Check sheet for the modelled part. Datum: model origin and axes. Units: mm. A direction names the side the tool comes from. Give positions to 0.01 mm unless a question says otherwise; leave off trailing zeros. Loops run counter-clockwise (first coordinate to the right, second up) from the corner with the lowest first, then second, coordinate; pieces in that order, holes last. Notation, with made-up numbers: (28.5, -6) - (82.5, -6) arc R16 ccw to (82.5, 8) - close; hole circle Ø3 at (-34.5, -0.75). An arc over 180 degrees is marked (long way). Answer in a Markdown table with one row per item. Add a question column.
(1) Thickness scan on L1, parallel to Y at x = 53.2, z = 1.15; L2, parallel to Z at x = 58.5, y = -27.4; L3, parallel to Z at x = 52.5, y = -24.5. Record the ranges inside material, lowest first.
(2) Sectioned sample at D-D on y = -27. Enter the section's corners in (x, z).
(3) Sectioned sample at A-A on x = 53.2. Enter the section's corners in (y, z), then the cut area to 3 significant figures.
(4) Set-up check for faces 4 (the face through (54, -10, 3)), 5 (the face through (55.2, 4, 8)), 6 (the face through (58, -20.162, 31)), 7 (the face through (59, -24.661, 40)): record each of +Z, -Z, +X, -X, +Y, -Y from which the full face is reachable in a straight line by a thin tool's end or side.
(5) Draft check along X on faces 1 (the face through (55.2, -22, 52)), 2 (the face through (58.242, -7.389, 47.625)), 3 (the face through (54.38, 2.98, 1.48)). Enter one of: released by +X, released by -X, zero draft, split by the parting line, or undercut.
(6) Go/stop test with flat-tipped pins: P1, Ø6, axis at x = 57, z = 77, coming from the -Y side; P2, Ø6.5, axis at x = 58, z = 27.5, coming from the +Y side; P3, Ø0.8, axis at y = 4, z = 10, coming from the -X side. Record where each tip stops, or that it passes through.
(7) Sectioned sample at C-C on z = 44. Enter the section's corners in (x, y).
(8) Sectioned sample at B-B on x = 58.5. Enter the section's corners in (y, z), then the cut area to 3 significant figures.
Autodesk Inventor part; units mm, degrees
ref_plane "Płaszczyzna konstrukcyjna3" through (-147.5, -30.65, -16.2) normal (0, 1, 0) x (0, 0, 1)
ref_plane "YZ Plane" through (0, 0, 0) normal (1, 0, 0) x (0, 1, 0)
ref_plane "XZ Plane" through (0, 0, 0) normal (0, 1, 0) x (-1, 0, 0)
ref_plane "Płaszczyzna konstrukcyjna2" through (0, 0, 0) normal (0, 0, 1) x (1, 0, 0)
sketch "Szkic2" plane through (0, 0, 0) normal (0, 0, 1) x (1, 0, 0)
  circle A0 centre (53.2, -19.05) radius 2
  circle A1 centre (53.2, 1.9) radius 2
  line L0 (61.2, -24.6614) -> (49.2, -24.6614)
  line L1 (49.2, -24.6614) -> (49.2, 5.9)
  line L2 (49.2, 5.9) -> (61.2, 5.9)
  line L3 (61.2, 5.9) -> (61.2, -24.6614)
  line L4 (60, -30.65) -> (57, -30.65)
  point P0 (0, 0)
  dimension "d0" = 4
  dimension "d1" = 4
  dimension "d2" = 12
  dimension "d3" = 30.5614
extrude "Wyciągnięcie proste1" add sketch "Szkic2" along normal blind 87.3125 contours A0 | A1 | L0 L1 L2 L3
sketch "Szkic3" plane through (49.2, -24.6614, 0) normal (0, -1, 0) x (1, 0, 0)
  circle A0 centre (9.3, 84.9) radius 1.5
  circle A1 centre (9.3, 84.9) radius 1.45
  point P0 (-49.2, 0)
  dimension "d6" = 2.9
extrude "Wyciągnięcie proste2" cut sketch "Szkic3" against normal blind 10 contours A1
sketch "Szkic4" plane through (0, 0, 0) normal (0, 0, -1) x (-1, 0, 0)
  point P0 (0, 0)
sketch "Szkic6" plane through (61.2, -24.6614, 0) normal (1, 0, 0) x (0, 0, -1)
  point P0 (0, 24.6614)
sketch "Szkic5" plane through (0, 0, 0) normal (0, 0, -1) x (-1, 0, 0)
  circle A0 centre (-53.2, 1.9) radius 2
  circle A1 centre (-53.2, -19.05) radius 2
  circle A2 centre (-53.2, -19.05) radius 1.6
  circle A3 centre (-53.2, 1.9) radius 1.6
  point P0 (0, 0)
  dimension "d9" = 3.2
  dimension "d10" = 3.2
extrude "Wyciągnięcie proste3" cut sketch "Szkic5" against normal blind 6 contours A2 | A3
sketch "Szkic7" plane through (61.2, -24.6614, 0) normal (1, 0, 0) x (0, 0, -1)
  line L0 (-87.3125, 30.5614) -> (-87.3125, 0)
  line L1 (-87.3125, 4.3495) -> (-6.8101, 30.5614)
  line L2 (-57.6962, 10.3521) -> (-6.9288, 26.8822)
  line L3 (0, 28.1614) -> (-6, 28.1614)
  line L4 (-3, 24.0296) -> (-3, 7.4995)
  line L5 (-6, 4.4995) -> (-56.7674, 4.4995)
  line L6 (0, 30.5614) -> (-87.3125, 30.5614)
  arc A0 (-57.6962, 10.3521) -> (-56.7674, 4.4995) centre (-56.7674, 7.4995) ccw
  arc A1 (-6, 4.4995) -> (-3, 7.4995) centre (-6, 7.4995) ccw
  arc A2 (-3, 24.0296) -> (-6.9288, 26.8822) centre (-6, 24.0296) ccw
  point P0 (0, 24.6614)
  point P1 (-75.6708, 4.4995)
  point P2 (-3, 28.1614)
  point P3 (-3, 4.4995)
  dimension "d17" = 3
extrude "Wyciągnięcie proste4" cut sketch "Szkic7" against normal blind 14.7625
sketch "Szkic8" plane through (49.2, -24.6614, 0) normal (0, -1, 0) x (1, 0, 0)
  line L0 (0, 87.3125) -> (12, 87.3125)
  line L1 (0, 0) -> (0, 6.8101)
  line L2 (12, 0) -> (12, 87.3125)
  line L3 (0, 0) -> (0, 87.3125)
  line L4 (0, 0) -> (12, 0)
  line L5 (6, 87.3125) -> (6, 3)
  line L6 (12, 3) -> (0, 3)
  point P0 (-49.2, 0)
extrude "Wyciągnięcie proste5" cut sketch "Szkic8" against normal blind 30.6375 contours L0 L5 L6 L1 L3
sketch "Szkic9" plane through (49.2, -24.6614, 0) normal (0, -1, 0) x (1, 0, 0)
  line L0 (6, 87.3125) -> (6, 3)
  line L1 (12, 6.8101) -> (12, 87.3125)
  line L2 (6, 87.3125) -> (12, 87.3125)
  line L3 (12, 87.3125) -> (12, 81.8248)
  line L4 (12, 81.8248) -> (6, 81.8248)
  line L5 (6, 81.8248) -> (6, 87.3125)
  circle A0 centre (9.3, 84.9) radius 1.5
  point P0 (-49.2, 0)
ref_plane "Płaszczyzna konstrukcyjna3" through (-147.5, -30.65, -16.2) normal (0, 1, 0) x (0, 0, 1)
extrude "Wyciągnięcie proste6" add sketch "Szkic9" along normal up to surface (5.9886 mm away)
sketch "Szkic10" plane through (61.2, -17.1619, 3) normal (0, 0, 1) x (1, 0, 0)
  point P0 (-61.2, 17.1619)
sketch "Szkic11" plane through (61.2, -17.1619, 3) normal (0, 0, 1) x (1, 0, 0)
  circle A0 centre (-8, -1.8881) radius 1.6
  circle A1 centre (-8, 19.0619) radius 1.6
  circle A2 centre (-8, -1.8881) radius 1.6
  circle A3 centre (-8, -1.8881) radius 2.5
  circle A4 centre (-8, 19.0619) radius 2.5
  point P0 (-61.2, 17.1619)
  dimension "d20" = 5
extrude "Wyciągnięcie proste7" cut sketch "Szkic11" along normal blind 28.575 contours A0 | A1 | A3 | A4
fillet "Zaokrąglenie1" radius 3.175 2 edges at (49.2, 5.9, 1.5) (49.2, -24.6614, 1.5)
properties part number "wzmocnienie"
Reply:
| question | item | result |
|---|---|---|
| 1 | L1 | -24.66 to -20.65, -17.45 to 0.3, 3.5 to 5.9 |
| 1 | L2 | 81.82 to 83.4, 86.4 to 87.31 |
| 1 | L3 | 0 to 3 |
| 2 | outline | (55.2, 81.82) - (61.2, 81.82) - (61.2, 87.31) - (55.2, 87.31) - close; hole circle Ø3 at (58.5, 84.9) |
| 3 | outline | (-24.66, 0) - (-20.65, 0) - (-20.65, 3) - (-24.66, 3) - close; (-17.45, 0) - (0.3, 0) - (0.3, 3) - (-17.45, 3) - close; (3.5, 0) - (5.9, 0) - (5.9, 3) - (3.5, 3) - close |
| 3 | area | 72.5 mm^2 |
| 4 | face 4 | -X |
| 4 | face 5 | +Z, -X, +Y, -Y |
| 4 | face 6 | +X, -X |
| 4 | face 7 | -Z, +X, -X, -Y |
| 5 | face 1 | released by -X |
| 5 | face 2 | zero draft |
| 5 | face 3 | undercut |
| 6 | P1 | y = -24.66 |
| 6 | P2 | y = 0.22 |
| 6 | P3 | x = 55.2 |
| 7 | outline | (55.2, -24.66) - (61.2, -24.66) - (61.2, -20.16) - (55.2, -20.16) - close; (55.2, -9.85) - (61.2, -9.85) - (61.2, -6.21) - (55.2, -6.21) - close |
| 8 | outline | (-30.65, 81.82) - (-24.66, 81.82) - (-24.66, 0) - (5.9, 0) - (5.9, 6.81) - (-19.05, 83.45) - (-24.66, 83.45) - (-24.66, 83.4) - (-30.65, 83.4) - close; (-30.65, 86.4) - (-24.66, 86.4) - (-24.66, 86.35) - (-20, 86.35) - (-20.31, 87.31) - (-30.65, 87.31) - close; hole (-20.16, 6) arc R3 ccw to (-17.16, 3) - (-0.63, 3) arc R3 ccw to (2.22, 6.93) - (-14.31, 57.7) arc R3 ccw to (-20.16, 56.77) - close |
| 8 | area | 803 mm^2 |
